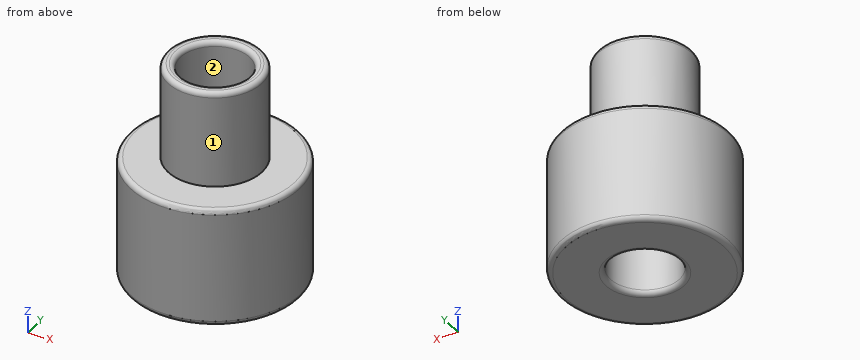
from build123d import *

# Parameters (mm, degrees)
F0_R     = 4.4
F1_DEPTH = 6.2
F2_R     = 2.45
F3_DEPTH = 5
F4_R     = 1.8034
F5_DEPTH = 11.201
F6_R     = 0.254


with BuildPart() as f1:
    # F0 (on Top) → F1 (new body)
    with BuildSketch(Plane.XY):
        Circle(F0_R)
    extrude(amount=F1_DEPTH)

    # F2 (on face) → F3 (join)
    with BuildSketch(Plane.XY.offset(6.2)):
        Circle(F2_R)
    extrude(amount=F3_DEPTH)

    # F4 (on face) → F5 (cut, through all)
    with BuildSketch(Plane(origin=(0, 0, 0), x_dir=(1, 0, 0), z_dir=(0, 0, -1))):
        Circle(F4_R)
    extrude(amount=-F5_DEPTH, mode=Mode.SUBTRACT)

    # F6
    f6_edges = [f1.edges().sort_by_distance(p)[0] for p in [
        (-2.45, 0, 11.2),
        (-1.8034, 0, 11.2),
        (-4.4, 0, 0),
        (-1.8034, 0, 0),
        (-4.4, 0, 6.2),
    ]]
    fillet(f6_edges, radius=F6_R)


solid = f1.part
Part model, mm, in its own coordinate system. Face numbers are marked on the shaded views. A direction names the side the tool comes from. Round coordinates to 2 decimals unless told otherwise and drop trailing zeros. Write each loop counter-clockwise with the first axis right and the second up, starting at its lowest first coordinate (ties: lowest second). Pieces come first, ordered by that corner, then holes. Notation, with made-up numbers: M 79,62 L 112,62 A14 ccw 112,80 Z; hole C 89,-9.75 d3. An arc over 180 degrees is marked long. Return JSON: item names as keys, results as strings. Group by question number.
(1) Which spindle directions (+Z, -Z, +X, -X, +Y, -Y) get a long thin tool onto all of the face, cutting with end or side? Do the marked faces 1 and 2. Say none if no direction does.
(2) Saw through at D-D on z = 8. Write the cut outline in (x, y).
(3) Saw through at C-C on z = 2. Write the cut outline in (x, y), then the cut area to 3 significant figures.
(4) Pin check, flat tips, straight feed: pin 1 Ø1 at (x, z) = (3.5, 3.5) entering from +Y; pin 2 Ø4 at (y, z) = (0.5, 3) entering from +X; pin 3 Ø1 at (y, z) = (3, 5.5) entering from -X. Stop position of each tip, or through.
(5) Saw through at A-A on x = 0. Write the cut outline in (y, z), then the cut area to 3 significant figures.
(6) Drill centre lines: probe 1 along Y at (x, z) = (0, 6.75); probe 2 along Z at (x, y) = (-3.5, 1.5); probe 3 along Y at (x, z) = (0, 4.5). Where is each one in solid material? Low to high.
Returned:
{
 "1": {"face 1": "+Z", "face 2": "+Z, -Z"},
 "2": {"outline": "C 0,0 d4.9; hole C 0,0 d3.61"},
 "3": {"outline": "C 0,0 d8.8; hole C 0,0 d3.61", "area": "50.6 mm²"},
 "4": {"pin 1": "y = 3.22", "pin 2": "x = 4.4", "pin 3": "x = -3.62"},
 "5": {"outline": "M -4.4,0.25 A0.25 ccw -4.15,0 L -2.06,0 A0.25 ccw -1.8,0.25 L -1.8,10.95 A0.25 ccw -2.06,11.2 L -2.2,11.2 A0.25 ccw -2.45,10.95 L -2.45,6.2 L -4.15,6.2 A0.25 ccw -4.4,5.95 Z; M 1.8,0.25 A0.25 ccw 2.06,0 L 4.15,0 A0.25 ccw 4.4,0.25 L 4.4,5.95 A0.25 ccw 4.15,6.2 L 2.45,6.2 L 2.45,10.95 A0.25 ccw 2.2,11.2 L 2.06,11.2 A0.25 ccw 1.8,10.95 Z", "area": "38.5 mm²"},
 "6": {"probe 1": "-2.45 to -1.8, 1.8 to 2.45", "probe 2": "0 to 6.2", "probe 3": "-4.4 to -1.8, 1.8 to 4.4"}
}
